Could you check a few things on this model? Use its own coordinates, in mm. Coordinates: 2 decimals unless noted, no trailing zeros. Order: outer loops, then holes, each group sorted by start corner. A loop starts at its lowest first (then second) coordinate and runs counter-clockwise, first axis right, second up. Notation, with made-up numbers: (-27.75, 56.5) - (24.25, 56.5) arc R23 cw to (24.25, 69.5) - close; hole circle Ø5 at (0, 36.25). An arc over 180 degrees is marked (long way). Answer as a JSON object with one key per item and string values. Group by question number.
(1) Imagine slicing it at D-D, the plane x = -22. Write out the boundary of the cut face in (y, z).
(2) Please list where these lines run through material, in increasing order: probe 1 along Y at (x, z) = (-11.5, 0.15); probe 2 along X at (y, z) = (-6.5, 0.65); probe 3 along X at (y, z) = (2, 0.3).
(3) Imagine slicing it at B-B, the plane x = -4.5. Write out the boundary of the cut face in (y, z), and give its area (3 significant figures).
(4) Imagine slicing it at A-A, the plane y = -2.75. Write out the boundary of the cut face in (x, z).
from build123d import *

# Parameters (mm, degrees)
SKETCH1_W      = 15.4432
SKETCH1_H      = 7.62
EXTRUDE1_DEPTH = 0.762
FILLET1_R      = 3.175


with BuildPart() as part:
    # Sketch1 → Extrude1 (new body)
    with BuildSketch(Plane.XY):
        Polygon((3.709668038, 4.91810583), (-11.793104343, 5.188707728), (-27.295876724, 4.91810583), (-27.295876724, -15.876690374), (-11.793104343, -16.147292272), (3.709668038, -15.876690374), align=None)
        with Locations((-11.793104343, -5.479292272)):
            Rectangle(SKETCH1_W, SKETCH1_H, mode=Mode.SUBTRACT)
    extrude(amount=EXTRUDE1_DEPTH)

    # Fillet1
    fillet1_edges = [part.edges().sort_by_distance(p)[0] for p in [
        (3.709668038, -15.876690374, 0.381),
        (-27.295876724, -15.876690374, 0.381),
        (-27.295876724, 4.91810583, 0.381),
        (3.709668038, 4.91810583, 0.381),
    ]]
    fillet(fillet1_edges, radius=FILLET1_R)


solid = part.part
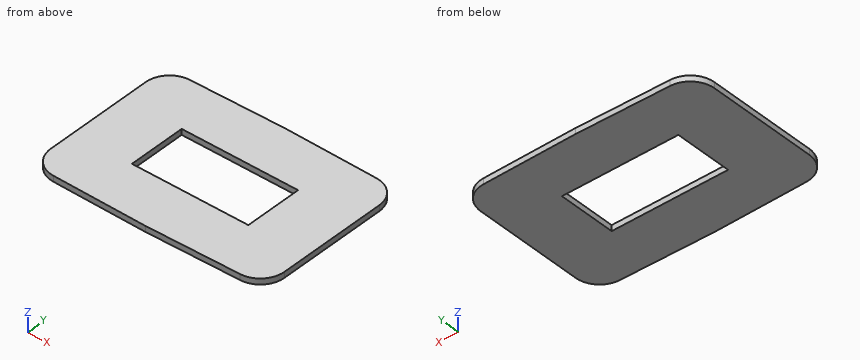
Result set:
{
 "1": {"outline": "(-15.97, 0) - (5.01, 0) - (5.01, 0.76) - (-15.97, 0.76) - close"},
 "2": {"probe 1": "y = -16.14 to -9.29, -1.67 to 5.18", "probe 2": "x = -27.3 to -19.51, -4.07 to 3.71", "probe 3": "x = -27.29 to 3.7"},
 "3": {"outline": "(-16.02, 0) - (-9.29, 0) - (-9.29, 0.76) - (-16.02, 0.76) - close; (-1.67, 0) - (5.06, 0) - (5.06, 0.76) - (-1.67, 0.76) - close", "area": "10.3 mm^2"},
 "4": {"outline": "(-27.3, 0) - (-19.51, 0) - (-19.51, 0.76) - (-27.3, 0.76) - close; (-4.07, 0) - (3.71, 0) - (3.71, 0.76) - (-4.07, 0.76) - close"}
}
